from build123d import *

# Parameters (mm, degrees)
SKETCH1_W                                      = 35
SKETCH1_H                                      = 35
BOSS_EXTRUDE1_DEPTH                            = 3
SKETCH3_W                                      = 25
SKETCH3_H                                      = 25
CUT_EXTRUDE2_DEPTH                             = 25.929901725
SKETCH4_W                                      = 45
SKETCH4_H                                      = 45
SKETCH4_W_2                                    = 30
SKETCH4_H_2                                    = 30
BOSS_EXTRUDE2_DEPTH                            = 1
CHAMFER2_SIZE                                  = 1
CSK_FOR_M2_FLAT_HEAD_MACHINE_SCREW1_AT_2_COUNT = 2
CSK_FOR_M2_FLAT_HEAD_MACHINE_SCREW1_AT_2_PITCH = 29
CSK_FOR_M2_FLAT_HEAD_MACHINE_SCREW1_AT_3_COUNT = 2
CSK_FOR_M2_FLAT_HEAD_MACHINE_SCREW1_AT_3_PITCH = 41.012193309
CSK_FOR_M2_FLAT_HEAD_MACHINE_SCREW1_AT_4_COUNT = 2
CSK_FOR_M2_FLAT_HEAD_MACHINE_SCREW1_AT_4_PITCH = 29
CSK_FOR_M2_FLAT_HEAD_MACHINE_SCREW1_AT_5_COUNT = 2
CSK_FOR_M2_FLAT_HEAD_MACHINE_SCREW1_AT_5_PITCH = 20.506096654
CUT_EXTRUDE3_START                             = 10
SKETCH7_R                                      = 2.2
CUT_EXTRUDE3_DEPTH                             = 10


with BuildPart() as part:
    # Sketch1 → Boss-Extrude1 (new body)
    with BuildSketch(Plane(origin=(0, 0, 0), x_dir=(1, 0, 0), z_dir=(0, 1, 0))):
        Rectangle(SKETCH1_W, SKETCH1_H)
    extrude(amount=BOSS_EXTRUDE1_DEPTH)

    # Sketch3 → Cut-Extrude2 (cut, through all)
    with BuildSketch(Plane(origin=(0, 3, 0), x_dir=(1, 0, 0), z_dir=(0, 1, 0))):
        Rectangle(SKETCH3_W, SKETCH3_H)
    extrude(amount=-CUT_EXTRUDE2_DEPTH, mode=Mode.SUBTRACT)

    # Sketch4 → Boss-Extrude2 (add)
    with BuildSketch(Plane(origin=(0, 3, 0), x_dir=(1, 0, 0), z_dir=(0, 1, 0))):
        Rectangle(SKETCH4_W, SKETCH4_H)
        Rectangle(SKETCH4_W_2, SKETCH4_H_2, mode=Mode.SUBTRACT)
    extrude(amount=BOSS_EXTRUDE2_DEPTH)

    # Chamfer2
    chamfer2_edges = [part.edges().sort_by_distance(p)[0] for p in [
        (0, 4, -15),
        (-15, 4, 0),
        (0, 4, 15),
        (15, 4, 0),
        (0, 4, 22.5),
        (-22.5, 4, 0),
        (0, 4, -22.5),
        (22.5, 4, 0),
    ]]
    chamfer(chamfer2_edges, length=CHAMFER2_SIZE - 0.0001)  # a hair under: the kernel refuses the full size

    # Sketch5 → CSK for M2 Flat Head Machine Screw1 (revolve, cut)
    with BuildSketch(Plane(origin=(14.5, 3, -14.5), x_dir=(0, 0, 1), z_dir=(1, 0, 0))):
        Polygon((0, 0), (0, 20.660946681), (1.1, 20), (1.1, 1.25), (2.2, 0.15), (2.2, 0), align=None)
    csk_for_m2_flat_head_machine_screw1 = revolve(axis=Axis((14.5, 9.35, -14.5), (0, -1, 0)), mode=Mode.SUBTRACT)

    # CSK for M2 Flat Head Machine Screw1 at 2: CSK for M2 Flat Head Machine Screw1 ×2
    with Locations(*[(0, 0, i * CSK_FOR_M2_FLAT_HEAD_MACHINE_SCREW1_AT_2_PITCH) for i in range(1, CSK_FOR_M2_FLAT_HEAD_MACHINE_SCREW1_AT_2_COUNT)]):
        add(csk_for_m2_flat_head_machine_screw1, mode=Mode.SUBTRACT)

    # CSK for M2 Flat Head Machine Screw1 at 3: CSK for M2 Flat Head Machine Screw1 ×2
    with Locations(*[Vector(-0.70710678118655, 0, 0.7071067811865451) * (i * CSK_FOR_M2_FLAT_HEAD_MACHINE_SCREW1_AT_3_PITCH) for i in range(1, CSK_FOR_M2_FLAT_HEAD_MACHINE_SCREW1_AT_3_COUNT)]):
        add(csk_for_m2_flat_head_machine_screw1, mode=Mode.SUBTRACT)

    # CSK for M2 Flat Head Machine Screw1 at 4: CSK for M2 Flat Head Machine Screw1 ×2
    with Locations(*[(-i * CSK_FOR_M2_FLAT_HEAD_MACHINE_SCREW1_AT_4_PITCH, 0, 0) for i in range(1, CSK_FOR_M2_FLAT_HEAD_MACHINE_SCREW1_AT_4_COUNT)]):
        add(csk_for_m2_flat_head_machine_screw1, mode=Mode.SUBTRACT)

    # CSK for M2 Flat Head Machine Screw1 at 5: CSK for M2 Flat Head Machine Screw1 ×2
    with Locations(*[Vector(-0.7071067811865493, 0, 0.7071067811865457) * (i * CSK_FOR_M2_FLAT_HEAD_MACHINE_SCREW1_AT_5_PITCH) for i in range(1, CSK_FOR_M2_FLAT_HEAD_MACHINE_SCREW1_AT_5_COUNT)]):
        add(csk_for_m2_flat_head_machine_screw1, mode=Mode.SUBTRACT)

    # Sketch7 → Cut-Extrude3 (cut)
    with BuildSketch(Plane(origin=(0, 3, 0), x_dir=(1, 0, 0), z_dir=(0, 1, 0)).offset(CUT_EXTRUDE3_START)):
        with Locations(Location((14.5, 14.5, 0), (0, 0, 270))):
            Circle(SKETCH7_R)
        with Locations(Location((14.5, -14.5, 0), (0, 0, 270))):
            Circle(SKETCH7_R)
        with Locations(Location((-14.5, -14.5, 0), (0, 0, 270))):
            Circle(SKETCH7_R)
        with Locations(Location((-14.5, 14.5, 0), (0, 0, 270))):
            Circle(SKETCH7_R)
    extrude(amount=-CUT_EXTRUDE3_DEPTH, mode=Mode.SUBTRACT)


solid = part.part
The listing builds one solid part. Answer for the finished solid, in the listing's coordinates (mm). A direction names the side the tool comes from. Give positions to 0.01 mm unless a question says otherwise; leave off trailing zeros. Write each loop counter-clockwise with the first axis right and the second up, starting at its lowest first coordinate (ties: lowest second). Pieces come first, ordered by that corner, then holes.
Item 1: Section B-B, the plane y = 0.85 is taken. Write down the section's boundary in (x, z), plus the area to 3 significant figures.
Item 2: Flat-ended cylindrical pins translate along their axes: P1, Ø9, axis at x = 1.5, z = 7, coming from the +Y side; P2, Ø1.5, axis at x = -3.5, y = 3.5, coming from the -Z side; P3, Ø3.5, axis at x = 14.5, z = -14.5, coming from the -Y side; P4, Ø1.5, axis at x = -1.5, y = 1, coming from the -Z side. Find the tip coordinate at first contact, or state that the pin passes through.
Item 3: Find the intervals of material crossed by line 1 along Z through (x, y) = (14.5, 2.95); line 2 along X through (y, z) = (0.5, 14.5), in increasing order.
Item 4: Determine the mould class of faces 6 (the flat face through (22, 3.5, 0.3)), 7 (the flat face through (-15.5, 3.5, 0.2)), 8 (the flat face through (0, 1, 17.5)), 9 (the cylindrical face through (15.574, 0.887, -14.738)) for opening direction Z: released by +Z, released by -Z, zero draft, split by the parting line, or undercut.
Item 5: Which of the six approach directions +Z, -Z, +X, -X, +Y, -Y give full straight-line access (tool end or side, diameter ignored) to faces 1 (the flat face through (-17.5, 1, 0)), 2 (the flat face through (-13, 3, 0)), 3 (the flat face through (0, 2, -12.5)), 4 (the flat face through (-22, 3.5, 0.3)), 5 (the flat face through (19, 4, 0))?
Completed:
1. outline: (-17.5, -17.5) - (17.5, -17.5) - (17.5, 17.5) - (-17.5, 17.5) - close; hole circle Ø2.2 at (-14.5, -14.5); hole circle Ø2.2 at (-14.5, 14.5); hole (-12.5, -12.5) - (12.5, -12.5) - (12.5, 12.5) - (-12.5, 12.5) - close; hole circle Ø2.2 at (14.5, -14.5); hole circle Ø2.2 at (14.5, 14.5)
1. area: 585 mm2
2. P1: passes through
2. P2: stops at z = -22.5
2. P3: stops at y = 0
2. P4: stops at z = -17.5
3. line 1: z = -17.5 to -16.7, -12.3 to 12.3, 16.7 to 17.5
3. line 2: x = -17.5 to -15.6, -13.4 to 13.4, 15.6 to 17.5
4. face 6: zero draft
4. face 7: undercut
4. face 8: released by +Z
4. face 9: undercut
5. face 1: +Z, -Z, -X, -Y
5. face 2: +Y
5. face 3: +Y, -Y
5. face 4: +Z, -Z, -X, +Y
5. face 5: +Z, -Z, +X, -X, +Y
